Geometry check sheet. Reference: the model listing, model coordinates, mm. Face numbers are marked on the shaded views. A direction names the side the tool comes from. Coordinates: 2 decimals unless noted, no trailing zeros. Write each loop counter-clockwise with the first axis right and the second up, starting at its lowest first coordinate (ties: lowest second). Pieces come first, ordered by that corner, then holes. Notation, with made-up numbers: (65, 63) - (93, 63) arc R27 ccw to (93, 101) - close; hole circle Ø9 at (-36, 57). An arc over 180 degrees is marked (long way). Answer as a JSON object with one key per item and string values. Group by question number.
from build123d import *

# Parameters (mm, degrees)
SKETCH1_W                      = 60
SKETCH1_H                      = 50
BOSS_EXTRUDE1_DEPTH            = 8
FILLET1_R                      = 10
CBORE_FOR_M6_SHCS1_D           = 6.6
CBORE_FOR_M6_SHCS1_DEPTH       = 10.1
CBORE_FOR_M6_SHCS1_CBORE_D     = 11
CBORE_FOR_M6_SHCS1_CBORE_DEPTH = 6
CBORE_FOR_M6_SHCS1_TIP         = 1.982840043
SKETCH4_W                      = 16.7
SKETCH4_H                      = 14
BOSS_EXTRUDE2_DEPTH            = 5
M5_CLEARANCE_HOLE1_D           = 5.3
M5_CLEARANCE_HOLE1_DEPTH       = 10
M5_CLEARANCE_HOLE1_TIP         = 1.59228064
BOSS_EXTRUDE3_DEPTH            = 2
FILLET2_R                      = 2
SKETCH8_R                      = 6.12
CUT_EXTRUDE1_DEPTH             = 59.386642308


with BuildPart() as part:
    # Sketch1 → Boss-Extrude1 (new body)
    with BuildSketch(Plane(origin=(0, 0, 0), x_dir=(1, 0, 0), z_dir=(0, 1, 0))):
        Rectangle(SKETCH1_W, SKETCH1_H)
    extrude(amount=BOSS_EXTRUDE1_DEPTH)

    # Fillet1
    fillet1_edges = [part.edges().sort_by_distance(p)[0] for p in [
        (30, 4, 25),
        (-30, 4, 25),
        (-30, 4, -25),
        (30, 4, -25),
    ]]
    fillet(fillet1_edges, radius=FILLET1_R)

    # CBORE for M6 SHCS1
    with Locations(Plane(origin=(0, 8, 0), x_dir=(1, 0, 0), z_dir=(0, 1, 0))):
        with Locations((-20, 15), (-20, -15), (20, -15), (20, 15)):
            CounterBoreHole(CBORE_FOR_M6_SHCS1_D / 2, CBORE_FOR_M6_SHCS1_CBORE_D / 2, CBORE_FOR_M6_SHCS1_CBORE_DEPTH, depth=CBORE_FOR_M6_SHCS1_DEPTH)
            with Locations((0, 0, -(CBORE_FOR_M6_SHCS1_DEPTH + CBORE_FOR_M6_SHCS1_TIP / 2))):  # 118° drill point
                Cone(0, CBORE_FOR_M6_SHCS1_D / 2, CBORE_FOR_M6_SHCS1_TIP, mode=Mode.SUBTRACT)

    # Sketch4 → Boss-Extrude2 (add)
    with BuildSketch(Plane(origin=(0, 0, -25), x_dir=(-1, 0, 0), z_dir=(0, 0, -1))):
        with Locations((0, 15)):
            Rectangle(SKETCH4_W, SKETCH4_H)
    extrude(amount=-BOSS_EXTRUDE2_DEPTH)

    # M5 Clearance Hole1
    with Locations(Plane.XY.offset(-20)):
        with Locations((0, 15.65)):
            Hole(M5_CLEARANCE_HOLE1_D / 2, depth=M5_CLEARANCE_HOLE1_DEPTH)
            with Locations((0, 0, -(M5_CLEARANCE_HOLE1_DEPTH + M5_CLEARANCE_HOLE1_TIP / 2))):  # 118° drill point
                Cone(0, M5_CLEARANCE_HOLE1_D / 2, M5_CLEARANCE_HOLE1_TIP, mode=Mode.SUBTRACT)

    # Sketch7 → Boss-Extrude3 (add)
    with BuildSketch(Plane(origin=(8.35, 0, 0), x_dir=(0, 0, -1), z_dir=(1, 0, 0))):
        Polygon((20, 22), (6, 8), (25, 8), (25, 22), align=None)
    boss_extrude3 = extrude(amount=BOSS_EXTRUDE3_DEPTH)

    # Mirror1: Boss-Extrude3 across plane
    add(boss_extrude3.mirror(Plane(origin=(0, 0, 0), x_dir=(0, 0, 1), z_dir=(1, 0, 0))))

    # Fillet2
    fillet2_edges = [part.edges().sort_by_distance(p)[0] for p in [
        (-10.35, 8, -15.5),
        (-9.35, 8, -6),
        (-8.35, 8, -13),
        (0, 8, -20),
        (8.35, 15, -20),
        (-8.35, 15, -20),
        (8.35, 8, -13),
        (9.35, 8, -6),
        (10.35, 8, -15.5),
    ]]
    fillet(fillet2_edges, radius=FILLET2_R)

    # Sketch8 → Cut-Extrude1 (cut, through all)
    with BuildSketch(Plane.XY.offset(-20)):
        with Locations((0, 15.65)):
            Circle(SKETCH8_R)
    extrude(amount=CUT_EXTRUDE1_DEPTH, mode=Mode.SUBTRACT)


solid = part.part
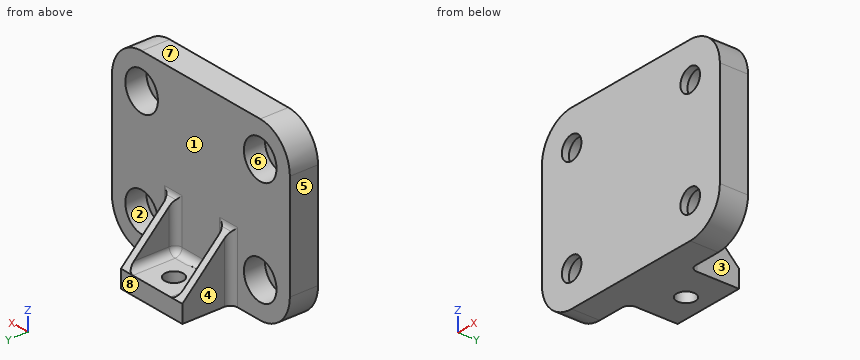
(1) Draft check along Z on the marked faces 6, 7 and 8. Enter one of: +Z half, -Z half, draft (parallel to the pull), parting line (faces both ways), or undercut.
(2) Section check D-D (z = 10.5). Record the cut outline in (x, y).
(3) Set-up check for the marked faces 1, 2, 3, 4 and 5: record each of +Z, -Z, +X, -X, +Y, -Y from which the full face is reachable in a straight line by a thin tool's end or side.
(4) Section check C-C (x = -18.5). Record the cut outline in (y, z).
(5) Gauge pin test, flat ends, axial feed: pin 1 (3.5 mm diameter, centred on x = -19.5, z = -14, fed in from +Y); pin 2 (6 mm diameter, centred on x = -11, y = 18.5, fed in from +Z); pin 3 (12 mm diameter, centred on x = 18.5, z = -15.5, fed in from +Y); pin 4 (12 mm diameter, centred on x = 23.5, z = 11.5, fed in from -Y). Record the tip position at first contact, or that the pin passes through.
(6) Section check A-A (y = 15.65). Record the cut outline in (x, z), and give its area (3 significant figures).
(7) Material ranges on L1, parallel to Z at x = 20, y = 6.35; L2, parallel to X at y = 0.55, z = -15; L3, parallel to X at y = 5.25, z = -13, recorded low to high. Write a range as [from, to].
(8) Section check B-B (y = 2.75). Record the cut outline in (x, z), and give its area (3 significant figures).
Conclusion:
{
 "1": {"face 6": "undercut", "face 7": "+Z half", "face 8": "draft"},
 "2": {"outline": "(-30, 0) - (30, 0) - (30, 8) - (23.16, 8) - (23.16, 2) - (16.84, 2) - (16.84, 8) - (-16.84, 8) - (-16.84, 2) - (-23.16, 2) - (-23.16, 8) - (-30, 8) - close"},
 "3": {"face 1": "+Z, +Y", "face 2": "+Y", "face 3": "+Z, -Z, +X, +Y", "face 4": "+Z, -Z, -X, +Y", "face 5": "+Z, -Z, -X, +Y, -Y"},
 "4": {"outline": "(0, -25) - (8, -25) - (8, -20.29) - (2, -20.29) - (2, -17.94) - (0, -17.94) - close; (0, -12.06) - (2, -12.06) - (2, -9.71) - (8, -9.71) - (8, 9.71) - (2, 9.71) - (2, 12.06) - (0, 12.06) - close; (0, 17.94) - (2, 17.94) - (2, 20.29) - (8, 20.29) - (8, 25) - (0, 25) - close"},
 "5": {"pin 1": "passes through", "pin 2": "stops at z = -13.57", "pin 3": "stops at y = 8", "pin 4": "stops at y = 0"},
 "6": {"outline": "(-10.35, -25) - (-2.65, -25) - (-2.65, -20) - (-6.35, -20) arc R2 cw to (-8.35, -18) - (-8.35, -13.65) - (-10.35, -13.65) - close; (2.65, -25) - (10.35, -25) - (10.35, -13.65) - (8.35, -13.65) - (8.35, -18) arc R2 cw to (6.35, -20) - (2.65, -20) - close", "area": "104 mm^2"},
 "7": {"L1": "z = [-25, -20.5], [-9.5, 9.5], [20.5, 25]", "L2": "x = [-30, -23.3], [-16.7, 16.7], [23.3, 30]", "L3": "x = [-30, -25.12], [-14.88, 14.88], [25.12, 30]"},
 "8": {"outline": "(-30, -15) arc R10 ccw to (-20, -25) - (20, -25) arc R10 ccw to (30, -15) - (30, 15) arc R10 ccw to (20, 25) - (-20, 25) arc R10 ccw to (-30, 15) - close; hole circle Ø11 at (-20, -15); hole circle Ø11 at (-20, 15); hole circle Ø11 at (20, -15); hole circle Ø11 at (20, 15)", "area": "2,530 mm^2"}
}
